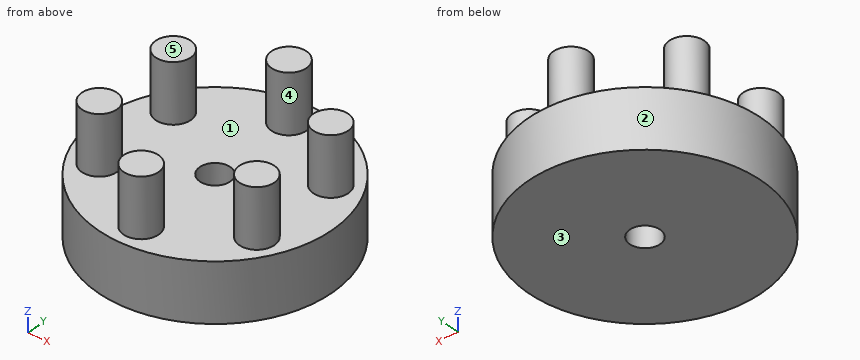
from build123d import *

# Parameters (mm, degrees)
F0_R     = 25.4
F2_DEPTH = 12.7
F1_R     = 3.81
F3_DEPTH = 25.4
F4_R     = 3.302
F5_DEPTH = 25.4


with BuildPart() as f2:
    # F0 (on Top) → F2 (new body)
    with BuildSketch(Plane.XY):
        Circle(F0_R)
    extrude(amount=F2_DEPTH)

    # F1 (on Top) → F3 (join)
    with BuildSketch(Plane.XY):
        with Locations((0, 19.503224)):
            Circle(F1_R)
        with Locations((-16.890287, 9.751612)):
            Circle(F1_R)
        with Locations((-16.890287, -9.751612)):
            Circle(F1_R)
        with Locations((0, -19.503224)):
            Circle(F1_R)
        with Locations((16.890287, -9.751612)):
            Circle(F1_R)
        with Locations((16.890287, 9.751612)):
            Circle(F1_R)
    extrude(amount=F3_DEPTH)

    # F4 (on Top) → F5 (cut)
    with BuildSketch(Plane.XY):
        Circle(F4_R)
    extrude(amount=F5_DEPTH, mode=Mode.SUBTRACT)


solid = f2.part
Can you work these out from the model? Positions are in its coordinate system, mm. Face numbers are marked on the shaded views. A direction names the side the tool comes from. Give positions to 0.01 mm unless a question says otherwise; leave off trailing zeros. Loops run counter-clockwise (first coordinate to the right, second up) from the corner with the lowest first, then second, coordinate; pieces in that order, holes last. Notation, with made-up numbers: (29.25, 89) -> (71.25, 89) arc R34 cw to (71.25, 127) -> close; hole circle Ø6 at (73, 28.25). An arc over 180 degrees is marked (long way). Write item = value, one per line.
1) Suppose I cut it at C-C on z = 23.5. Write out the boundary of the cut face in (x, y), then the cut area to 3 significant figures.
Check result:
outline = circle Ø7.62 at (-16.89, -9.75); circle Ø7.62 at (-16.89, 9.75); circle Ø7.62 at (0, -19.5); circle Ø7.62 at (0, 19.5); circle Ø7.62 at (16.89, -9.75); circle Ø7.62 at (16.89, 9.75)
area = 274 mm2
2) For the marked faces 4 and 5, which set-ups out of +Z, -Z, +X, -X, +Y, -Y let a thin tool reach every point of the face, with its end or its side?
Check result:
face_4 = +Z
face_5 = +Z, +X, -X, +Y, -Y
3) Suppose I cut it at D-D on x = -19. Write out the boundary of the cut face in (y, z), then the cut area to 3 significant figures.
Check result:
outline = (-16.86, 0) -> (16.86, 0) -> (16.86, 12.7) -> (12.92, 12.7) -> (12.92, 25.4) -> (6.58, 25.4) -> (6.58, 12.7) -> (-6.58, 12.7) -> (-6.58, 25.4) -> (-12.92, 25.4) -> (-12.92, 12.7) -> (-16.86, 12.7) -> close
area = 589 mm2
4) Thinking about a two-plate mould opening in X: for the marked faces 1, 2 and 3, which applies, released by +X, released by -X, zero draft, split by the parting line, or undercut?
Check result:
face_1 = undercut
face_2 = split by the parting line
face_3 = zero draft
5) Suppose I cut it at B-B on y = 2.5. Write out the boundary of the cut face in (x, z).
Check result:
outline = (-25.28, 0) -> (-2.16, 0) -> (-2.16, 12.7) -> (-25.28, 12.7) -> close; (2.16, 0) -> (25.28, 0) -> (25.28, 12.7) -> (2.16, 12.7) -> close
6) Will these pins go through, and if not, where does the flat tip stop? pin 1 (10 mm diameter, centred on y = -10.5, z = 5, fed in from -X); pin 2 (2 mm diameter, centred on x = 18, z = 11.5, fed in from +Y); pin 3 (1.5 mm diameter, centred on x = 2, y = 5.5, fed in from +Z).
Check result:
pin_1 = -24.8
pin_2 = 18.87
pin_3 = 12.7
7) I need wall thicknesses on L1, parallel to X at y = 10, z = 16.75; L2, parallel to Y at x = 0, z = 6.5; L3, parallel to Z at x = 7, y = 21. Which ranges of each line are inside material? Lowest first, please. Write a range as from..to.
Check result:
L1 = -20.69..-13.09, 13.09..20.69
L2 = -25.4..-3.3, 3.3..25.4
L3 = 0..12.7
8) Suppose I cut it at A-A on x = 0. Write out the boundary of the cut face in (y, z), then the cut area to 3 significant figures.
Check result:
outline = (-25.4, 0) -> (-3.3, 0) -> (-3.3, 12.7) -> (-15.69, 12.7) -> (-15.69, 25.4) -> (-23.31, 25.4) -> (-23.31, 12.7) -> (-25.4, 12.7) -> close; (3.3, 0) -> (25.4, 0) -> (25.4, 12.7) -> (23.31, 12.7) -> (23.31, 25.4) -> (15.69, 25.4) -> (15.69, 12.7) -> (3.3, 12.7) -> close
area = 755 mm2
